from build123d import *

# Parameters (mm, degrees)
SKETCH_1_W             = 150
SKETCH_1_H             = 36
EXTRUDE_2_DEPTH        = 6
SKETCH_6_W             = 10
SKETCH_6_H             = 6
EXTRUDE_4_DEPTH        = 4
PATTERN_LINEAR_1_COUNT = 6
PATTERN_LINEAR_1_PITCH = 25
SKETCH_8_W             = 5
SKETCH_8_H             = 6
SKETCH_8_W_2           = 4.995224333
CUT_EXTRUDE_3_DEPTH    = 6
SKETCH_11_W            = 4.504775667
SKETCH_11_H            = 6
SKETCH_11_W_2          = 4.5
CUT_EXTRUDE_4_DEPTH    = 6
SKETCH_12_W            = 35.2
SKETCH_12_H            = 25.2
CUT_EXTRUDE_5_DEPTH    = 155.376163963
SKETCH_14_W            = 15
SKETCH_14_H            = 6
SKETCH_14_W_2          = 10
CUT_EXTRUDE_6_DEPTH    = 4
SKETCH_15_W            = 15
SKETCH_15_H            = 6
EXTRUDE_5_DEPTH        = 1
PATTERN_LINEAR_2_COUNT = 5
PATTERN_LINEAR_2_PITCH = 25
SKETCH_16_W            = 15
SKETCH_16_H            = 6
EXTRUDE_6_DEPTH        = 1
SKETCH_17_W            = 10
SKETCH_17_H            = 6
EXTRUDE_7_DEPTH        = 1
SKETCH_18_W            = 15
SKETCH_18_H            = 6
EXTRUDE_8_DEPTH        = 1


with BuildPart() as part:
    # Эскиз1 → Бобышка-Вытянуть2 (new body)
    with BuildSketch(Plane(origin=(0, 0, 0), x_dir=(1, 0, 0), z_dir=(0, 1, 0))):
        with Locations((75, -18)):
            Rectangle(SKETCH_1_W, SKETCH_1_H)
    extrude(amount=EXTRUDE_2_DEPTH)

    # Эскиз6 → Бобышка-Вытянуть4 (add)
    with BuildSketch(Plane(origin=(0, 0, 0), x_dir=(-1, 0, 0), z_dir=(0, 0, -1))):
        with Locations((-5, 3)):
            Rectangle(SKETCH_6_W, SKETCH_6_H)
    extrude_4 = extrude(amount=EXTRUDE_4_DEPTH)

    # Линейный массив1: Бобышка-Вытянуть4 ×6
    with Locations(*[(i * PATTERN_LINEAR_1_PITCH, 0, 0) for i in range(1, PATTERN_LINEAR_1_COUNT)]):
        add(extrude_4)

    # Эскиз8 → Вырез-Вытянуть3 (cut)
    with BuildSketch(Plane.ZY):
        with Locations((6.5, 3)):
            Rectangle(SKETCH_8_W, SKETCH_8_H)
        with Locations((16, 3)):
            Rectangle(SKETCH_8_W, SKETCH_8_H)
        with Locations((25.502387834, 3)):
            Rectangle(SKETCH_8_W_2, SKETCH_8_H)
    extrude(amount=-CUT_EXTRUDE_3_DEPTH, mode=Mode.SUBTRACT)

    # Эскиз11 → Вырез-Вытянуть4 (cut)
    with BuildSketch(Plane(origin=(150, 0, 0), x_dir=(0, 0, -1), z_dir=(1, 0, 0))):
        with Locations((-20.752387834, 3)):
            Rectangle(SKETCH_11_W, SKETCH_11_H)
        with Locations((-11.25, 3)):
            Rectangle(SKETCH_11_W_2, SKETCH_11_H)
    extrude(amount=-CUT_EXTRUDE_4_DEPTH, mode=Mode.SUBTRACT)

    # Эскиз12 → Вырез-Вытянуть5 (cut, through all)
    with BuildSketch(Plane(origin=(0, 6, 0), x_dir=(1, 0, 0), z_dir=(0, 1, 0))):
        with Locations((67.6, -19.4)):
            Rectangle(SKETCH_12_W, SKETCH_12_H)
    extrude(amount=-CUT_EXTRUDE_5_DEPTH, mode=Mode.SUBTRACT)

    # Эскиз14 → Вырез-Вытянуть6 (cut)
    with BuildSketch(Plane.XY.offset(36)):
        with Locations((17.5, 3)):
            Rectangle(SKETCH_14_W, SKETCH_14_H)
        with Locations((130, 3)):
            Rectangle(SKETCH_14_W_2, SKETCH_14_H)
    extrude(amount=-CUT_EXTRUDE_6_DEPTH, mode=Mode.SUBTRACT)

    # Эскиз15 → Бобышка-Вытянуть5 (add)
    with BuildSketch(Plane(origin=(0, 0, 0), x_dir=(-1, 0, 0), z_dir=(0, 0, -1))):
        with Locations((-17.5, 3)):
            Rectangle(SKETCH_15_W, SKETCH_15_H)
    extrude_5 = extrude(amount=EXTRUDE_5_DEPTH)

    # Линейный массив2: Бобышка-Вытянуть5 ×5
    with Locations(*[(i * PATTERN_LINEAR_2_PITCH, 0, 0) for i in range(1, PATTERN_LINEAR_2_COUNT)]):
        add(extrude_5)

    # Эскиз16 → Бобышка-Вытянуть6 (add)
    with BuildSketch(Plane(origin=(0, 0, 0), x_dir=(-1, 0, 0), z_dir=(0, 0, -1))):
        with Locations((-142.5, 3)):
            Rectangle(SKETCH_16_W, SKETCH_16_H)
    extrude(amount=EXTRUDE_6_DEPTH)

    # Эскиз17 → Бобышка-Вытянуть7 (add)
    with BuildSketch(Plane.XY.offset(32)):
        with Locations((130, 3)):
            Rectangle(SKETCH_17_W, SKETCH_17_H)
    extrude(amount=EXTRUDE_7_DEPTH)

    # Эскиз18 → Бобышка-Вытянуть8 (add)
    with BuildSketch(Plane.XY.offset(32)):
        with Locations((17.5, 3)):
            Rectangle(SKETCH_18_W, SKETCH_18_H)
    extrude(amount=EXTRUDE_8_DEPTH)


solid = part.part
Model file for the job. Use its own axes, mm. A direction names the side the tool comes from. Round coordinates to 2 decimals unless told otherwise and drop trailing zeros. Order: outer loops, then holes, each group sorted by start corner. A loop starts at its lowest first (then second) coordinate and runs counter-clockwise, first axis right, second up.
(1) Pin check, flat tips, straight feed: pin 1 (1.8 mm diameter, centred on x = 115, y = 3.5, fed in from -Z); pin 2 (0.9 mm diameter, centred on y = 2.5, z = -3, fed in from +X); pin 3 (1.5 mm diameter, centred on x = 127.5, y = 5.5, fed in from +Z). Stop position of each tip, or through.
(2) Pull direction X, two halves, no side cores. Call faces 5 (the face through (85, 3, -2)), 6 (the face through (0, 3, 21)), 7 (the face through (30, 3, -4)): released by +X, released by -X, zero draft, split by the parting line, or undercut.
(3) Drill centre lines: line 1 (X direction, y = 0.7, z = -2); line 2 (X direction, y = 2.5, z = 29.5); line 3 (Z direction, x = 57, y = 0.95). Where is each one in solid material? Low to high.
(4) Band-saw the part on B-B (x = 21.5). List the corners of the cut face in (y, z).
(5) Band-saw the part on C-C (x = 40.5). List the corners of the cut face in (y, z).
(6) 3-axis set-ups, long thin cutter, end or side, ignore diameter. For faces 1 (the face through (50, 3, 20)), 2 (the face through (3, 3, 13.5)), 3 (the face through (18, 3, -1)), 4 (the face through (144, 3, 21)): which of +Z, -Z, +X, -X, +Y, -Y reach the whole face in a straight line?
(7) Band-saw the part on A-A (x = 66). List the corners of the cut face in (y, z), then the cut area to 3 significant figures.
Verdict:
1. pin 1: stops at z = -1
1. pin 2: stops at x = 135
1. pin 3: stops at z = 33
2. face 5: undercut
2. face 6: released by -X
2. face 7: zero draft
3. line 1: x = 0 to 10, 25 to 35, 50 to 60, 75 to 85, 100 to 110, 125 to 135
3. line 2: x = 0 to 50, 85.2 to 150
3. line 3: z = -4 to 6.8, 32 to 36
4. outline: (0, -1) - (6, -1) - (6, 33) - (0, 33) - close
5. outline: (0, -1) - (6, -1) - (6, 36) - (0, 36) - close
6. face 1: +Y, -Y
6. face 2: -X, +Y, -Y
6. face 3: -Z, +Y, -Y
6. face 4: +X, +Y, -Y
7. outline: (0, -1) - (6, -1) - (6, 6.8) - (0, 6.8) - close; (0, 32) - (6, 32) - (6, 36) - (0, 36) - close
7. area: 70.8 mm2
